Check sheet for the modelled part. Datum: model origin and axes. Units: mm. Round coordinates to 2 decimals unless told otherwise and drop trailing zeros. Write each loop counter-clockwise with the first axis right and the second up, starting at its lowest first coordinate (ties: lowest second). Pieces come first, ordered by that corner, then holes. Notation, with made-up numbers: (87.25, -28) -> (142.25, -28) arc R20 cw to (142.25, -18) -> close; hole circle Ø4 at (53.25, 56). An arc over 180 degrees is marked (long way). Use one line per item in the form item = value. Start each with the question number.
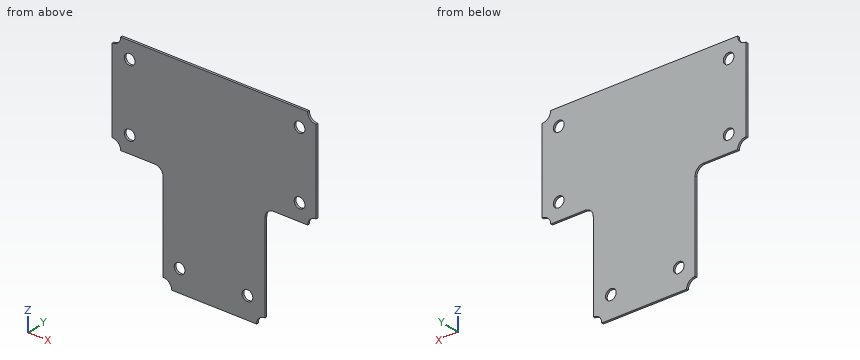
```python
from build123d import *

# Parameters (mm, degrees)
F0_R     = 8.001
F1_DEPTH = 3.175


with BuildPart() as f1:
    # F0 (on Front) → F1 (new body)
    with BuildSketch(Plane.XZ):
        with BuildLine():
            ThreePointArc((153.411418, 63.5), (144.431162, 67.219744), (140.711418, 76.2))
            Line((140.711418, 76.2), (-138.688582, 76.2))
            ThreePointArc((-138.688582, 76.2), (-142.408326, 67.219744), (-151.388582, 63.5))
            Line((-151.388582, 63.5), (-151.388582, -63.5))
            ThreePointArc((-151.388582, -63.5), (-142.408326, -67.219744), (-138.688582, -76.2))
            Line((-138.688582, -76.2), (-87.888582, -76.2))
            ThreePointArc((-87.888582, -76.2), (-78.908326, -79.919744), (-75.188582, -88.9))
            Line((-75.188582, -88.9), (-75.188582, -223.730639))
            ThreePointArc((-75.188582, -223.730639), (-66.208326, -227.450383), (-62.488582, -236.430639))
            Line((-62.488582, -236.430639), (64.380207, -236.430639))
            ThreePointArc((64.380207, -236.430639), (68.099951, -227.450383), (77.080207, -223.730639))
            Line((77.080207, -223.730639), (77.080207, -88.9))
            ThreePointArc((77.080207, -88.9), (80.799951, -79.919744), (89.780207, -76.2))
            Line((89.780207, -76.2), (140.711418, -76.2))
            ThreePointArc((140.711418, -76.2), (144.431162, -67.219744), (153.411418, -63.5))
            Line((153.411418, -63.5), (153.411418, 63.5))
        make_face()
        with Locations((-50.668789, -203.2)):
            Circle(F0_R, mode=Mode.SUBTRACT)
        with Locations((50.8, -203.2)):
            Circle(F0_R, mode=Mode.SUBTRACT)
        with Locations((-125.302818, -50.8)):
            Circle(F0_R, mode=Mode.SUBTRACT)
        with Locations((-125.302818, 50.8)):
            Circle(F0_R, mode=Mode.SUBTRACT)
        with Locations((128.697182, -50.8)):
            Circle(F0_R, mode=Mode.SUBTRACT)
        with Locations((128.697182, 50.8)):
            Circle(F0_R, mode=Mode.SUBTRACT)
    extrude(amount=F1_DEPTH)


solid = f1.part
```
1. Depth check by flat-ended pin: pin 1 (1 mm diameter, centred on x = 110, y = -2, fed in from -Z); pin 2 (1.6 mm diameter, centred on y = -1.5, z = -149, fed in from +X). Enter the tip coordinate at first touch or a pass-through.
2. Scan lines: probe 1 along Z at (x, y) = (128, -2.6); probe 2 along X at (y, z) = (-2.7, -207); probe 3 along X at (y, z) = (-0.25, -56). Record each from-to range of solid material in increasing order.
3. Sectioned sample at A-A (x = 50.8). Enter the section's corners in (y, z) (3 decimals).
4. Sectioned sample at B-B (z = -50.8). Enter the section's corners in (x, y) (3 decimals).
5. Sectioned sample at D-D (z = -203.2). Enter the section's corners in (x, y) (3 decimals), and give its area (3 significant figures).
6. Sectioned sample at C-C (y = -2.6). Enter the section's corners in (x, z), and give its area (3 significant figures).
Returned:
q1.pin_1 = -76.2
q1.pin_2 = 77.08
q2.probe_1 = -76.2 to -58.77, -42.83 to 42.83, 58.77 to 76.2
q2.probe_2 = -75.19 to -57.71, -43.63 to 43.76, 57.84 to 77.08
q2.probe_3 = -151.39 to -131.38, -119.22 to 122.62, 134.78 to 153.41
q3.outline = (-3.175, -236.431) -> (0, -236.431) -> (0, -211.201) -> (-3.175, -211.201) -> close; (-3.175, -195.199) -> (0, -195.199) -> (0, 76.2) -> (-3.175, 76.2) -> close
q4.outline = (-151.389, -3.175) -> (-133.304, -3.175) -> (-133.304, 0) -> (-151.389, 0) -> close; (-117.302, -3.175) -> (120.696, -3.175) -> (120.696, 0) -> (-117.302, 0) -> close; (136.698, -3.175) -> (153.411, -3.175) -> (153.411, 0) -> (136.698, 0) -> close
q5.outline = (-75.189, -3.175) -> (-58.67, -3.175) -> (-58.67, 0) -> (-75.189, 0) -> close; (-42.668, -3.175) -> (42.799, -3.175) -> (42.799, 0) -> (-42.668, 0) -> close; (58.801, -3.175) -> (77.08, -3.175) -> (77.08, 0) -> (58.801, 0) -> close
q5.area = 382 mm^2
q6.outline = (-151.39, -63.5) arc R12.7 cw to (-138.69, -76.2) -> (-87.89, -76.2) arc R12.7 cw to (-75.19, -88.9) -> (-75.19, -223.73) arc R12.7 cw to (-62.49, -236.43) -> (64.38, -236.43) arc R12.7 cw to (77.08, -223.73) -> (77.08, -88.9) arc R12.7 cw to (89.78, -76.2) -> (140.71, -76.2) arc R12.7 cw to (153.41, -63.5) -> (153.41, 63.5) arc R12.7 cw to (140.71, 76.2) -> (-138.69, 76.2) arc R12.7 cw to (-151.39, 63.5) -> close; hole circle Ø16 at (-125.3, -50.8); hole circle Ø16 at (-125.3, 50.8); hole circle Ø16 at (-50.67, -203.2); hole circle Ø16 at (50.8, -203.2); hole circle Ø16 at (128.7, -50.8); hole circle Ø16 at (128.7, 50.8)
q6.area = 69,000 mm^2
